The model under review builds one solid part; all positions refer to its coordinate system, in mm. A direction names the side the tool comes from. Coordinates: 2 decimals unless noted, no trailing zeros. Loops run counter-clockwise (first coordinate to the right, second up) from the corner with the lowest first, then second, coordinate; pieces in that order, holes last. Notation, with made-up numbers: (11.5, -17) - (55.5, -17) arc R29 ccw to (55.5, 16) - close; hole circle Ø3 at (20.25, 61.25). An arc over 180 degrees is marked (long way). One line per item, written item: value. Start each with the question number.
1. Insertion check: P1, Ø9, axis at y = 28.35, z = 0, coming from the +X side; P2, Ø24, axis at y = -39.04, z = 38.91, coming from the -X side; P3, Ø5, axis at x = 10, z = 38.5, coming from the -Y side; P4, Ø4.5, axis at x = 3, y = 4.5, coming from the -Z side. Each pin has a flat end and moves straight along its axis. Give the tip position at first contact, or say it passes through.
2. We need section B-B, the plane z = 0. Give the boundary of the cut face in (x, y).
3. To check wall thickness, follow line 1 (Y direction, x = -1.5, z = 17.5); line 2 (Z direction, x = 26, y = -34.5); line 3 (Y direction, x = 2, z = 21). State the ranges of each line that lie inside material, in increasing order.
4. We need section C-C, the plane y = -6.5. Give the boundary of the cut face in (x, z), then the cut area to 3 significant figures.
5. We need section D-D, the plane x = -12.5. Give the boundary of the cut face in (y, z).
6. We need section A-A, the plane x = 5. Give the boundary of the cut face in (y, z).
7. Mouldability with a two-part tool opening along Z and no side actions: class faces 4 (the face through (17.2, -72.13, -42.59)), 5 (the face through (7, 6, 5.576)), 6 (the face through (37.477, -31, -15)) as +Z half, -Z half, draft (parallel to the pull), parting line (faces both ways), or undercut.
8. For faces 1 (the face through (-22.523, -10, -20)), 2 (the face through (7, 6, -3.763)), 3 (the face through (-2.523, 35, 31)), list the 3-axis set-ups (+Z, -Z, +X, -X, +Y, -Y) from which the entire face can be reached by the end or side of a thin tool; tool diameter is ignored.
from build123d import *

# Parameters (mm, degrees)
CUT_EXTRUDE1_DEPTH = 61
SKETCH3_R          = 7.5
CUT_EXTRUDE2_DEPTH = 21
CIRPATTERN1_COUNT  = 3


with BuildPart() as part:
    # Sketch1 → Revolve1 (revolve)
    with BuildSketch(Plane.XY):
        Polygon((-22.523252325, 13.422459893), (-22.523252325, -16.577540107), (37.476747675, -16.577540107), (37.476747675, 53.422459893), (-2.523252325, 53.422459893), (-2.523252325, 43.422459893), (17.476747675, 43.422459893), (17.476747675, 13.422459893), align=None)
    revolve(axis=Axis((-22.523252325, -16.577540107, 0), (1, 0, 0)))

    # Sketch2 → Cut-Extrude1 (cut, through all)
    with BuildSketch(Plane.ZY.offset(22.523252325)):
        with BuildLine():
            Line((-3.763166571, 3.06523407), (-3.763166571, 8.354397525))
            Line((-3.763166571, 8.354397525), (5.575592602, 8.354397525))
            Line((5.575592602, 8.354397525), (5.575592602, 2.62956189))
            ThreePointArc((5.575592602, 2.62956189), (-0.932027141, -36.555811439), (-3.763166571, 3.06523407))
        make_face()
    extrude(amount=-CUT_EXTRUDE1_DEPTH, mode=Mode.SUBTRACT)

    # Sketch3 → Cut-Extrude2 (cut, through all)
    with BuildSketch(Plane.ZY.offset(-17.476747675)):
        with Locations((0, 28.354397525)):
            Circle(SKETCH3_R)
    cut_extrude2 = extrude(amount=-CUT_EXTRUDE2_DEPTH, mode=Mode.SUBTRACT)

    # CirPattern1: Cut-Extrude2 ×3 about axis
    cirpattern1_axis = Axis((0, -16.577540107, 0), (1, 0, 0))
    for i in range(1, CIRPATTERN1_COUNT):
        add(cut_extrude2.rotate(cirpattern1_axis, i * 360 / CIRPATTERN1_COUNT), mode=Mode.SUBTRACT)


solid = part.part
Findings below:
1. P1: through
1. P2: x = 17.48
1. P3: y = -76.61
1. P4: z = -67.42
2. outline: (-22.52, -46.58) - (17.48, -46.58) - (17.48, -76.58) - (-2.52, -76.58) - (-2.52, -86.58) - (37.48, -86.58) - (37.48, -36.58) - (-22.52, -36.58) - close; (-22.52, 8.35) - (37.48, 8.35) - (37.48, 20.85) - (17.48, 20.85) - (17.48, 13.42) - (-22.52, 13.42) - close; (-2.52, 43.42) - (17.48, 43.42) - (17.48, 35.85) - (37.48, 35.85) - (37.48, 53.42) - (-2.52, 53.42) - close
3. line 1: -84.35 to -73.97, -40.94 to -26.26, -6.9 to 7.79, 40.81 to 51.2
3. line 2: -67.67 to -44.88, -32.95 to -8.88, 8.88 to 32.95, 44.88 to 67.67
3. line 3: -83.35 to -72.78, -38 to 4.85, 39.63 to 50.2
4. outline: (-22.52, -28.26) - (17.48, -28.26) - (17.48, -59.15) - (-2.52, -59.15) - (-2.52, -69.27) - (37.48, -69.27) - (37.48, -17.28) - (-22.52, -17.28) - close; (-22.52, 17.28) - (37.48, 17.28) - (37.48, 69.27) - (-2.52, 69.27) - (-2.52, 59.15) - (17.48, 59.15) - (17.48, 28.26) - (-22.52, 28.26) - close
4. area: 3,360 mm2
5. outline: circle Ø60 at (-16.58, 0); hole (2.63, 5.58) arc R20 ccw (long way) to (3.07, -3.76) - (8.35, -3.76) - (8.35, 5.58) - close
6. outline: circle Ø140 at (-16.58, 0); circle Ø60 at (-16.58, 0); hole circle Ø120 at (-16.58, 0); hole (2.63, 5.58) arc R20 ccw (long way) to (3.07, -3.76) - (8.35, -3.76) - (8.35, 5.58) - close
7. face 4: parting line
7. face 5: undercut
7. face 6: draft
8. face 1: +Z, -Z, -X, +Y, -Y
8. face 2: +X, -X
8. face 3: -X
